from build123d import *

# Parameters (mm, degrees)
SKETCH1_W         = 210
SKETCH1_H         = 210
MAINEXTRUDE_DEPTH = 4
SKETCH1_6_R       = 1.5
SCREWHOLES_DEPTH  = 4
ROUNDEDCORNERS_R  = 10
SKETCH3_R         = 7
TRENCH_DEPTH      = 4


with BuildPart() as part:
    # Sketch1 → MainExtrude (new body)
    with BuildSketch(Plane(origin=(0, 0, 0), x_dir=(1, 0, 0), z_dir=(0, 1, 0))):
        Rectangle(SKETCH1_W, SKETCH1_H)
    extrude(amount=MAINEXTRUDE_DEPTH)

    # Sketch1<6> → ScrewHoles (cut)
    with BuildSketch(Plane(origin=(0, 0, 0), x_dir=(1, 0, 0), z_dir=(0, 1, 0))):
        with Locations((-99.833273811, 99.833273811)):
            Circle(SKETCH1_6_R)
        with Locations((-99.833273811, -99.833273811)):
            Circle(SKETCH1_6_R)
        with Locations((99.833273811, -99.833273811)):
            Circle(SKETCH1_6_R)
        with Locations((99.833273811, 99.833273811)):
            Circle(SKETCH1_6_R)
    extrude(amount=SCREWHOLES_DEPTH, mode=Mode.SUBTRACT)

    # RoundedCorners
    roundedcorners_edges = [part.edges().sort_by_distance(p)[0] for p in [
        (-105, 2, -105),
        (-105, 2, 105),
        (105, 2, 105),
        (105, 2, -105),
    ]]
    fillet(roundedcorners_edges, radius=ROUNDEDCORNERS_R)

    # Sketch3 → Trench (cut)
    with BuildSketch(Plane(origin=(0, 0, 0), x_dir=(1, 0, 0), z_dir=(0, 1, 0))):
        with Locations((-52.205723714, -65.868416485)):
            Circle(SKETCH3_R)
        Polygon((-38, 90), (-38, 30), (-90, 30), (-90, 20), (0, 20), (0, -40), (-80, -40), (-80, -10), (-30, -10), (-30, 0), (-90, 0), (-90, -50), (-15, -50), (-15, -90), (85, -90), (85, -30), (50, -30), (50, 10), (90, 10), (90, 70), (80, 70), (80, 20), (40, 20), (40, -30), (25, -30), (25, -40), (75, -40), (75, -80), (-5, -80), (-5, -50), (10, -50), (10, 30), (-28, 30), (-28, 90), align=None)
    extrude(amount=TRENCH_DEPTH, mode=Mode.SUBTRACT)


solid = part.part
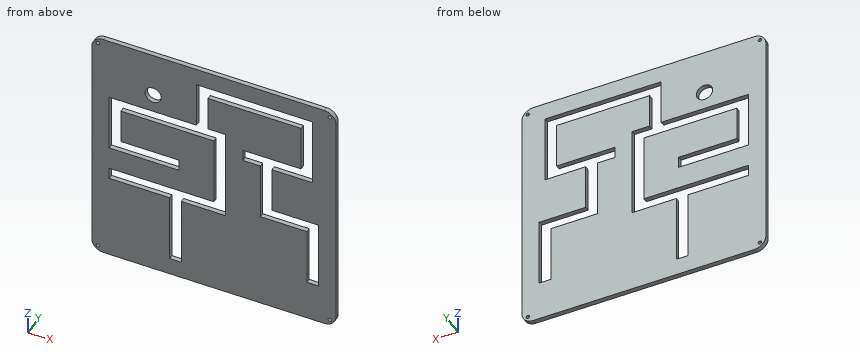
Can you work these out from the model? Positions are in its coordinate system, mm. Round coordinates to 2 decimals unless told otherwise and drop trailing zeros. Order: outer loops, then holes, each group sorted by start corner. A loop starts at its lowest first (then second) coordinate and runs counter-clockwise, first axis right, second up. Notation, with made-up numbers: (-4, 14) - (17, 14) arc R32 ccw to (17, 44) - close; hole circle Ø9 at (-11.5, -12.5). An arc over 180 degrees is marked (long way). Answer in a Markdown table with one row per item.
(1) Suppose I cut it at B-B, the plane z = -52. Please give me the cut outline in (x, y).
From the geometry:
| item | result |
|---|---|
| outline | (-105, 0) - (-38, 0) - (-38, 4) - (-105, 4) - close; (-28, 0) - (80, 0) - (80, 4) - (-28, 4) - close; (90, 0) - (105, 0) - (105, 4) - (90, 4) - close |
(2) Suppose I cut it at C-C, the plane y = 3. Count the separate pieces of the cut face and the enclosed holes in it, plus the area to 3 significant figures.
From the geometry:
| item | result |
|---|---|
| separate pieces | 1 |
| enclosed holes | 6 |
| area | 36,000 mm2 |
(3) Suppose I cut it at A-A, the plane x = 44.5. Please give me the cut outline in (y, z), plus the area to 3 significant figures.
From the geometry:
| item | result |
|---|---|
| outline | (0, -105) - (4, -105) - (4, -20) - (0, -20) - close; (0, 40) - (4, 40) - (4, 80) - (0, 80) - close; (0, 90) - (4, 90) - (4, 105) - (0, 105) - close |
| area | 560 mm2 |
(4) Please list where these lines run through material, in increasing order: L1, parallel to X at y = 0.75, z = 11; L2, parallel to Z at x = 44, y = 0.9; L3, parallel to Z at x = 78.5, y = 0.95. Write a range as from..to.
From the geometry:
| item | result |
|---|---|
| L1 | x = -105..-90, -80..0, 10..40, 50..105 |
| L2 | z = -105..-20, 40..80, 90..105 |
| L3 | z = -105..-20, -10..30, 90..105 |
